Autodesk Fusion 360 part; units mm, degrees
sketch "Sketch2" plane through (0, 0, 0) normal (0, 0, 1) x (1, 0, 0)
  circle A0 centre (0, 0) radius 9
  circle A1 centre (0, 0) radius 8
  circle A2 centre (0, 0) radius 2.1
  dimension "d10" = 16
  dimension "d26" = 4.2
extrude "Extrude3" add sketch "Sketch2" along normal blind 0.2 contours A1
sketch "Sketch3" plane through (0, 0, 0.2) normal (0, 0, 1) x (1, 0, 0)
  circle A0 centre (0, 0) radius 6.05
  circle A1 centre (0, 0) radius 8
  circle A2 centre (0, 0) radius 2.1
  dimension "d13" = 12.1
extrude "Extrude4" add sketch "Sketch3" along normal blind 8 contours A0
sketch "Sketch4" plane through (0, 0, 8.2) normal (0, 0, 1) x (1, 0, 0)
  circle A0 centre (0, 0) radius 6.05
  line L0 (-1.963, 3.4) -> (-3.926, 0)
  line L1 (-3.926, 0) -> (-1.963, -3.4)
  line L2 (-1.963, -3.4) -> (1.963, -3.4)
  line L3 (1.963, -3.4) -> (3.926, 0)
  line L4 (3.926, 0) -> (1.963, 3.4)
  line L5 (1.963, 3.4) -> (-1.963, 3.4)
  circle A1 centre (0, 0) radius 2.1
  dimension "d24" = 6.8
extrude "Extrude5" add sketch "Sketch4" along normal blind 10 contours L0 L1 L2 L3 L4 L5
The model under review builds one solid part; all positions refer to its coordinate system, in mm. A direction names the side the tool comes from. Round coordinates to 2 decimals unless told otherwise and drop trailing zeros. Write each loop counter-clockwise with the first axis right and the second up, starting at its lowest first coordinate (ties: lowest second). Pieces come first, ordered by that corner, then holes. Notation, with made-up numbers: (72, 63.5) -> (94, 63.5) arc R11 cw to (94, 72.5) -> close; hole circle Ø10 at (77.25, -37.5). An arc over 180 degrees is marked (long way). Answer as a JSON object with one key per item and string values.
1. Machinability: for faces 1 (the face through (2.958, 1.676, 13.13)), 2 (the face through (0, -3.4, 13)), 3 (the face through (0, 3.4, 13)), 4 (the face through (-2.931, 1.724, 13.13)), which of the approach directions +Z, -Z, +X, -X, +Y, -Y give a long, thin tool a straight path to every point of the face, cutting with its end or side? Answer none if there is none.
Results found:
{"face 1": "+Z, +X, +Y", "face 2": "+Z, +X, -X, -Y", "face 3": "+Z, +X, -X, +Y", "face 4": "+Z, -X, +Y"}
2. The part is to be moulded in two halves that separate along Y. For faces 5 (the face through (-2.958, -1.676, 13.13)), 6 (the face through (5.589, 2.317, 4.144)), 7 (the face through (3, -3, 8.2)), 8 (the face through (2.003, -0.631, 8.973)), say which applies: pulls with the +Y half, pulls with the -Y half, needs draft (parallel to the pull), parting line crosses it, or undercut.
Results found:
{"face 5": "pulls with the -Y half", "face 6": "parting line crosses it", "face 7": "needs draft", "face 8": "undercut"}
3. We need section C-C on y = -0.75. State the section outline as (x, z) points.
Results found:
{"outline": "(-7.96, 0) -> (-1.96, 0) -> (-1.96, 18.2) -> (-3.49, 18.2) -> (-3.49, 8.2) -> (-6, 8.2) -> (-6, 0.2) -> (-7.96, 0.2) -> close; (1.96, 0) -> (7.96, 0) -> (7.96, 0.2) -> (6, 0.2) -> (6, 8.2) -> (3.49, 8.2) -> (3.49, 18.2) -> (1.96, 18.2) -> close"}
4. We need section B-B on x = 0. State the section outline as (y, z) points.
Results found:
{"outline": "(-8, 0) -> (-2.1, 0) -> (-2.1, 18.2) -> (-3.4, 18.2) -> (-3.4, 8.2) -> (-6.05, 8.2) -> (-6.05, 0.2) -> (-8, 0.2) -> close; (2.1, 0) -> (8, 0) -> (8, 0.2) -> (6.05, 0.2) -> (6.05, 8.2) -> (3.4, 8.2) -> (3.4, 18.2) -> (2.1, 18.2) -> close"}
5. We need section D-D on y = -2.75. State the section outline as (x, z) points, and give its area (3 significant figures).
Results found:
{"outline": "(-7.51, 0) -> (7.51, 0) -> (7.51, 0.2) -> (5.39, 0.2) -> (5.39, 8.2) -> (2.34, 8.2) -> (2.34, 18.2) -> (-2.34, 18.2) -> (-2.34, 8.2) -> (-5.39, 8.2) -> (-5.39, 0.2) -> (-7.51, 0.2) -> close", "area": "136 mm^2"}
6. Clearance check with flat-ended pins moving along their axes: pin 1 (3 mm diameter, centred on x = 0, z = 14.5, fed in from +Y); pin 2 (5 mm diameter, centred on y = 5.5, z = 7.5, fed in from -X); pin 3 (1.2 mm diameter, centred on x = -0.5, z = 14, fed in from -Y). State where each tip first meets the part, or that it passes through.
Results found:
{"pin 1": "stops at y = 3.4", "pin 2": "stops at x = -5.25", "pin 3": "stops at y = -3.4"}
7. To check wall thickness, follow line 1 along Y through (x, z) = (0, 7.75); line 2 along Z through (x, y) = (2.5, 4); line 3 along Z through (x, y) = (5.5, 3.5). State the ranges of each line that lie inside material, in increasing order.
Results found:
{"line 1": "y = -6.05 to -2.1, 2.1 to 6.05", "line 2": "z = 0 to 8.2", "line 3": "z = 0 to 0.2"}
8. We need section A-A on z = 14. State the section outline as (x, y) points.
Results found:
{"outline": "(-3.93, 0) -> (-1.96, -3.4) -> (1.96, -3.4) -> (3.93, 0) -> (1.96, 3.4) -> (-1.96, 3.4) -> close; hole circle Ø4.2 at (0, 0)"}
